For this review, take the finished solid that the model builds, in its own axes (mm). Face numbers are marked on the shaded views. A direction names the side the tool comes from. Give positions to 0.01 mm unless a question says otherwise; leave off trailing zeros. Order: outer loops, then holes, each group sorted by start corner. A loop starts at its lowest first (then second) coordinate and runs counter-clockwise, first axis right, second up. Notation, with made-up numbers: (43.25, 3) -> (56.25, 3) arc R24 ccw to (56.25, 17) -> close; hole circle Ø1 at (39, 85.5). An arc over 180 degrees is marked (long way). Return JSON: item names as keys, results as strings. Group by question number.
1) For the marked faces 1 and 2, list the 3-axis set-ups (+Z, -Z, +X, -X, +Y, -Y) from which the entire face can be reached by the end or side of a thin tool; tool diameter is ignored.
2) Insertion check: P1, Ø9, axis at x = 34.5, z = 18, coming from the -Y side; P2, Ø24, axis at x = 11.5, z = 64, coming from the -Y side; P3, Ø6, axis at x = 69, z = 11.5, coming from the -Y side; P4, Ø12, axis at x = 57.5, z = 41, coming from the -Y side. Each pin has a flat end and moves straight along its axis. Give the tip position at first contact, or say it passes through.
3) Add section B-B (z = 64). Give the boundary of the cut face in (x, y).
4) The part is to be moulded in two halves that separate along Y. For the marked faces 3, 4, 5 and 6, say which applies: released by +Y, released by -Y, zero draft, split by the parting line, or undercut.
5) Add section A-A (x = 57.5). Give the boundary of the cut face in (y, z), then the cut area to 3 significant figures.
6) To check wall thickness, follow line 1 along X through (y, z) = (-1.15, 64); line 2 along Y through (x, z) = (70.5, 67); line 3 along Z through (x, y) = (67, -28.5). State the ranges of each line that lie inside material, in increasing order.
7) Add section D-D (z = 22). Give the boundary of the cut face in (x, y), then the cut area to 3 significant figures.
8) Add section C-C (x = 67.5). Give the boundary of the cut face in (y, z), then the cut area to 3 significant figures.
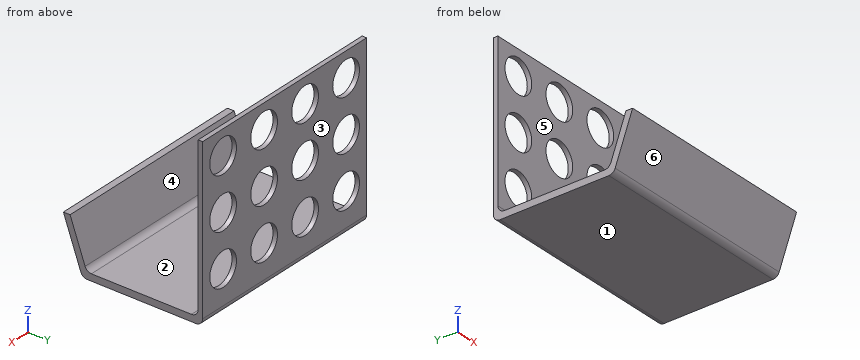
from build123d import *

# Parameters (mm, degrees)
PAD_DEPTH    = 92
SKETCH001_R  = 7.5
POCKET_DEPTH = 2


with BuildPart() as part:
    # Sketch → Pad (new body)
    with BuildSketch(Plane.YZ):
        with BuildLine():
            Line((0, 75), (0, 3))
            ThreePointArc((-3, 0), (-0.87868, 0.87868), (0, 3))
            Line((-3, 0), (-51.807467, 0))
            ThreePointArc((-54.626545, 1.97394), (-53.528196, 0.542544), (-51.807467, 0))
            Line((-54.626545, 1.97394), (-62.458589, 23.492317))
            Line((-62.458589, 23.492317), (-59.458589, 23.492317))
            Line((-52.718455, 4.97394), (-59.458589, 23.492317))
            ThreePointArc((-52.718455, 4.97394), (-51.620107, 3.542544), (-49.899377, 3))
            Line((-5, 3), (-49.899377, 3))
            ThreePointArc((-5, 3), (-2.87868, 3.87868), (-2, 6))
            Line((-2, 75), (-2, 6))
            Line((0, 75), (-2, 75))
        make_face()
    extrude(amount=PAD_DEPTH)

    # Sketch001 (on Face12 of Pad) → Pocket (cut)
    with BuildSketch(Plane(origin=(0, -2, 0), x_dir=(0, 0, -1), z_dir=(0, -1, 0))):
        with Locations((-64, 11.5)):
            Circle(SKETCH001_R)
        with Locations((-41, 11.5)):
            Circle(SKETCH001_R)
        with Locations((-18, 11.5)):
            Circle(SKETCH001_R)
        with Locations((-64, 34.5)):
            Circle(SKETCH001_R)
        with Locations((-41, 34.5)):
            Circle(SKETCH001_R)
        with Locations((-18, 34.5)):
            Circle(SKETCH001_R)
        with Locations((-64, 57.5)):
            Circle(SKETCH001_R)
        with Locations((-41, 57.5)):
            Circle(SKETCH001_R)
        with Locations((-18, 57.5)):
            Circle(SKETCH001_R)
        with Locations((-64, 80.5)):
            Circle(SKETCH001_R)
        with Locations((-41, 80.5)):
            Circle(SKETCH001_R)
        with Locations((-18, 80.5)):
            Circle(SKETCH001_R)
    extrude(amount=-POCKET_DEPTH, mode=Mode.SUBTRACT)


solid = part.part
Evaluation:
{
 "1": {"face 1": "-Z, +X, -X, +Y, -Y", "face 2": "+Z, +X, -X"},
 "2": {"P1": "y = -62.1", "P2": "y = -2", "P3": "y = -59.19", "P4": "through"},
 "3": {"outline": "(0, -2) -> (4, -2) -> (4, 0) -> (0, 0) -> close; (19, -2) -> (27, -2) -> (27, 0) -> (19, 0) -> close; (42, -2) -> (50, -2) -> (50, 0) -> (42, 0) -> close; (65, -2) -> (73, -2) -> (73, 0) -> (65, 0) -> close; (88, -2) -> (92, -2) -> (92, 0) -> (88, 0) -> close"},
 "4": {"face 3": "released by +Y", "face 4": "undercut", "face 5": "undercut", "face 6": "released by -Y"},
 "5": {"outline": "(-62.46, 23.49) -> (-54.63, 1.97) arc R3 ccw to (-51.81, 0) -> (-3, 0) arc R3 ccw to (0, 3) -> (0, 10.5) -> (-2, 10.5) -> (-2, 6) arc R3 cw to (-5, 3) -> (-49.9, 3) arc R3 cw to (-52.72, 4.97) -> (-59.46, 23.49) -> close; (-2, 25.5) -> (0, 25.5) -> (0, 33.5) -> (-2, 33.5) -> close; (-2, 48.5) -> (0, 48.5) -> (0, 56.5) -> (-2, 56.5) -> close; (-2, 71.5) -> (0, 71.5) -> (0, 75) -> (-2, 75) -> close", "area": "279 mm^2"},
 "6": {"line 1": "0 to 4, 19 to 27, 42 to 50, 65 to 73, 88 to 92", "line 2": "-2 to 0", "line 3": "0 to 3"},
 "7": {"outline": "(0, -61.92) -> (92, -61.92) -> (92, -58.92) -> (0, -58.92) -> close; (0, -2) -> (5.16, -2) -> (5.16, 0) -> (0, 0) -> close; (17.84, -2) -> (28.16, -2) -> (28.16, 0) -> (17.84, 0) -> close; (40.84, -2) -> (51.16, -2) -> (51.16, 0) -> (40.84, 0) -> close; (63.84, -2) -> (74.16, -2) -> (74.16, 0) -> (63.84, 0) -> close; (86.84, -2) -> (92, -2) -> (92, 0) -> (86.84, 0) -> close", "area": "358 mm^2"},
 "8": {"outline": "(-62.46, 23.49) -> (-54.63, 1.97) arc R3 ccw to (-51.81, 0) -> (-3, 0) arc R3 ccw to (0, 3) -> (0, 75) -> (-2, 75) -> (-2, 6) arc R3 cw to (-5, 3) -> (-49.9, 3) arc R3 cw to (-52.72, 4.97) -> (-59.46, 23.49) -> close", "area": "369 mm^2"}
}
